CAD build for the part. Positions are in the model's coordinates, mm. A direction names the side the tool comes from. Give positions to 0.01 mm unless a question says otherwise; leave off trailing zeros. Order: outer loops, then holes, each group sorted by start corner. A loop starts at its lowest first (then second) coordinate and runs counter-clockwise, first axis right, second up. Notation, with made-up numbers: M -34,77.5 L 0,77.5 A16 ccw 0,107.5 Z; hole C -16.5,44 d1. An arc over 180 degrees is marked long. Put each result on its own line as item: value. Start each with the question number.
1) Drill centre lines: line 1 (Y direction, x = 10.25, z = 14.5); line 2 (Z direction, x = 3.5, y = -39.5); line 3 (Z direction, x = 2, y = -9). Where is each one in solid material? Low to high. Write a range as [from, to].
2) Cut at D-D (x = 10.5). Write the cut outline in (y, z).
3) Cut at A-A (z = 0). Write the cut outline in (x, y), and give its area (3 significant figures).
4) Cut at C-C (x = 1.5). Give the number of separate pieces and of enclosed holes in the cut face, and give its area (3 significant figures).
5) Pin check, flat tips, straight feed: pin 1 (8 mm diameter, centred on y = 37.59, z = -32.97, fed in from +X); pin 2 (1 mm diameter, centred on x = 7.5, z = -6, fed in from -Y); pin 3 (4 mm diameter, centred on x = 10.5, y = 18.5, fed in from -Z). Stop position of each tip, or through.
6) Tool access for faces 1 (the face through (4, 0, -40)), 2 (the face through (6.59, -8.85, -51.9)), 3 (the face through (15.028, -8.178, -54.047)): list every direction of +Z, -Z, +X, -X, +Y, -Y with a clear straight run to the whole face (end or side of a thin tool).
```python
from build123d import *

# Parameters (mm, degrees)
SKETCH2_R          = 2.5
CUT_EXTRUDE1_DEPTH = 4
SKETCH3_R          = 3
CUT_EXTRUDE4_DEPTH = 87.539008545
SKETCH4_R          = 5.25
CUT_EXTRUDE5_DEPTH = 4


with BuildPart() as part:
    # Sketch1 → Revolve1 (revolve)
    with BuildSketch(Plane.XY, mode=Mode.PRIVATE) as revolve1_sk:
        Polygon((0, 60), (0, 33), (7, 33), (7, 26), (14, 26), (14, 23), (17, 23), (17, 60), align=None)
    revolve(revolve1_sk.sketch.rotate(Axis((0, 0, 0), (1, 0, 0)), 90), axis=Axis((0, 0, 0), (1, 0, 0)))

    # Sketch2 → Cut-Extrude1 (cut)
    with BuildSketch(Plane.ZY):
        with Locations((0, 40)):
            Circle(SKETCH2_R)
        with Locations((15.307337295, 36.9551813)):
            Circle(SKETCH2_R)
        with Locations((28.284271247, 28.284271247)):
            Circle(SKETCH2_R)
        with Locations((36.9551813, 15.307337295)):
            Circle(SKETCH2_R)
        with Locations((40, 0)):
            Circle(SKETCH2_R)
        with Locations((36.9551813, -15.307337295)):
            Circle(SKETCH2_R)
        with Locations((28.284271247, -28.284271247)):
            Circle(SKETCH2_R)
        with Locations((15.307337295, -36.9551813)):
            Circle(SKETCH2_R)
        with Locations((0, -40)):
            Circle(SKETCH2_R)
        with Locations((-15.307337295, -36.9551813)):
            Circle(SKETCH2_R)
        with Locations((-28.284271247, -28.284271247)):
            Circle(SKETCH2_R)
        with Locations((-36.9551813, -15.307337295)):
            Circle(SKETCH2_R)
        with Locations((-40, 0)):
            Circle(SKETCH2_R)
        with Locations((-36.9551813, 15.307337295)):
            Circle(SKETCH2_R)
        with Locations((-28.284271247, 28.284271247)):
            Circle(SKETCH2_R)
        with Locations((-15.307337295, 36.9551813)):
            Circle(SKETCH2_R)
    extrude(amount=-CUT_EXTRUDE1_DEPTH, mode=Mode.SUBTRACT)

    # Sketch3 → Cut-Extrude4 (cut, through all)
    with BuildSketch(Plane(origin=(17, 0, 0), x_dir=(0, 0, -1), z_dir=(1, 0, 0))):
        with Locations((49.03926402, -9.754516101)):
            Circle(SKETCH3_R)
        with Locations((16.071973265, -47.346506475)):
            Circle(SKETCH3_R)
        with Locations((-32.967290755, -37.591990374)):
            Circle(SKETCH3_R)
        with Locations((-49.03926402, 9.754516101)):
            Circle(SKETCH3_R)
        with Locations((-16.071973265, 47.346506475)):
            Circle(SKETCH3_R)
        with Locations((32.967290755, 37.591990374)):
            Circle(SKETCH3_R)
    extrude(amount=-CUT_EXTRUDE4_DEPTH, mode=Mode.SUBTRACT)

    # Sketch4 → Cut-Extrude5 (cut)
    with BuildSketch(Plane(origin=(17, 0, 0), x_dir=(0, 0, -1), z_dir=(1, 0, 0))):
        with Locations((32.967290755, 37.591990374)):
            Circle(SKETCH4_R)
        with Locations((49.03926402, -9.754516101)):
            Circle(SKETCH4_R)
        with Locations((16.071973265, -47.346506475)):
            Circle(SKETCH4_R)
        with Locations((-32.967290755, -37.591990374)):
            Circle(SKETCH4_R)
        with Locations((-49.03926402, 9.754516101)):
            Circle(SKETCH4_R)
        with Locations((-16.071973265, 47.346506475)):
            Circle(SKETCH4_R)
    extrude(amount=-CUT_EXTRUDE5_DEPTH, mode=Mode.SUBTRACT)


solid = part.part
```
Solution:
1. line 1: [-58.22, -21.58], [21.58, 44.79], [49.9, 58.22]
1. line 2: [-45.16, -2.45], [2.45, 30.65], [35.28, 45.16]
1. line 3: [-59.32, -51.94], [-46.14, -31.75], [31.75, 59.32]
2. outline: C 0,0 d120; hole C -47.35,-16.07 d6; hole C -37.59,32.97 d6; hole C 0,0 d52; hole C -9.75,-49.04 d6; hole C 9.75,49.04 d6; hole C 37.59,-32.97 d6; hole C 47.35,16.07 d6
3. outline: M 0,-60 L 17,-60 L 17,-23 L 14,-23 L 14,-26 L 7,-26 L 7,-33 L 0,-33 L 0,-37.5 L 4,-37.5 L 4,-42.5 L 0,-42.5 Z; M 0,33 L 7,33 L 7,26 L 14,26 L 14,23 L 17,23 L 17,60 L 0,60 L 0,42.5 L 4,42.5 L 4,37.5 L 0,37.5 Z
3. area: 1,040 mm²
4. separate pieces: 1
4. enclosed holes: 23
4. area: 7,400 mm²
5. pin 1: x = 13
5. pin 2: y = -59.75
5. pin 3: z = -57.69
6. face 1: -X
6. face 2: +X, -X
6. face 3: +X
